from build123d import *

# Parameters (mm, degrees)
SKETCH1_W           = 50.8
SKETCH1_H           = 34.925
BOSS_EXTRUDE1_DEPTH = 1.27
SKETCH2_W           = 1.27
SKETCH2_H           = 34.925
BOSS_EXTRUDE2_DEPTH = 36.83
SKETCH3_R           = 2.0828
CUT_EXTRUDE1_DEPTH  = 36.83
SKETCH4_R           = 2.0828
CUT_EXTRUDE2_DEPTH  = 36.83


with BuildPart() as part:
    # Sketch1 → Boss-Extrude1 (new body)
    with BuildSketch(Plane.XY):
        Rectangle(SKETCH1_W, SKETCH1_H)
    extrude(amount=BOSS_EXTRUDE1_DEPTH)

    # Sketch2 → Boss-Extrude2 (add)
    with BuildSketch(Plane.XY.offset(1.27)):
        with Locations((-24.765, 0)):
            Rectangle(SKETCH2_W, SKETCH2_H)
    extrude(amount=BOSS_EXTRUDE2_DEPTH)

    # Sketch3 → Cut-Extrude1 (cut)
    with BuildSketch(Plane(origin=(-24.13, 0, 0), x_dir=(0, 0, -1), z_dir=(1, 0, 0))):
        with Locations((-10.4775, 8.73125)):
            Circle(SKETCH3_R)
        with Locations((-28.8925, -8.73125)):
            Circle(SKETCH3_R)
    extrude(amount=-CUT_EXTRUDE1_DEPTH, mode=Mode.SUBTRACT)

    # Sketch4 → Cut-Extrude2 (cut)
    with BuildSketch(Plane.XY.offset(1.27)):
        with Locations((-11.7475, 8.47725)):
            Circle(SKETCH4_R)
        with Locations((13.0175, -8.73125)):
            Circle(SKETCH4_R)
    extrude(amount=-CUT_EXTRUDE2_DEPTH, mode=Mode.SUBTRACT)


solid = part.part
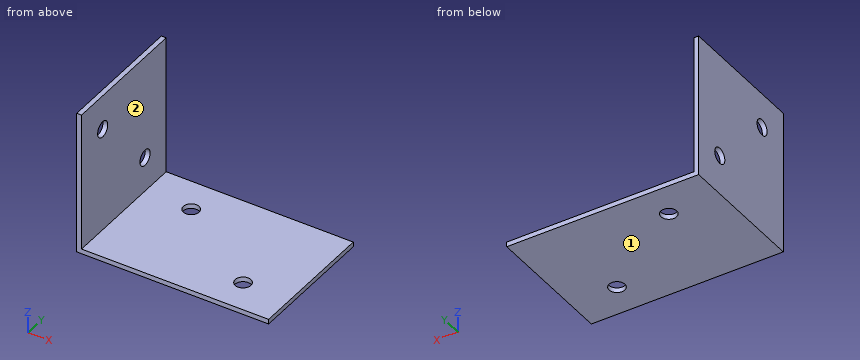
Model file for the job. Use its own axes, mm. Face numbers are marked on the shaded views. A direction names the side the tool comes from. Give positions to 0.01 mm unless a question says otherwise; leave off trailing zeros. Order: outer loops, then holes, each group sorted by start corner. A loop starts at its lowest first (then second) coordinate and runs counter-clockwise, first axis right, second up. Notation, with made-up numbers: (18, 74.5) - (72, 74.5) arc R24 ccw to (72, 107.5) - close; hole circle Ø2 at (20.5, 49.25). An arc over 180 degrees is marked (long way). One line per item, written item: value.
Item 1: Slice it at C-C (y = 5). List the corners of the cut face in (x, z).
Response values:
outline: (-25.4, 0) - (25.4, 0) - (25.4, 1.27) - (-24.13, 1.27) - (-24.13, 38.1) - (-25.4, 38.1) - close
Item 2: Slice it at D-D (z = 18). List the corners of the cut face in (x, y), then the cut area to 3 significant figures.
Response values:
outline: (-25.4, -17.46) - (-24.13, -17.46) - (-24.13, 17.46) - (-25.4, 17.46) - close
area: 44.4 mm2
Item 3: Pin check, flat tips, straight feed: pin 1 Ø3.5 at (y, z) = (-8.73, 28.89) entering from +X; pin 2 Ø12 at (x, z) = (8, 6.5) entering from +Y; pin 3 Ø2 at (x, y) = (-1, 8.5) entering from +Z; pin 4 Ø10.5 at (y, z) = (-2, 19.5) entering from +X. Stop position of each tip, or through.
Response values:
pin 1: through
pin 2: y = 17.46
pin 3: z = 1.27
pin 4: x = -24.13
Item 4: Slice it at B-B (x = 12). List the corners of the cut face in (y, z), then the cut area to 3 significant figures.
Response values:
outline: (-17.46, 0) - (-10.55, 0) - (-10.55, 1.27) - (-17.46, 1.27) - close; (-6.91, 0) - (17.46, 0) - (17.46, 1.27) - (-6.91, 1.27) - close
area: 39.7 mm2
Item 5: Tool access for the marked faces 1 and 2: list every direction of +Z, -Z, +X, -X, +Y, -Y with a clear straight run to the whole face (end or side of a thin tool).
Response values:
face 1: -Z, +X, -X, +Y, -Y
face 2: +Z, +X, +Y, -Y
Item 6: Slice it at A-A (z = 29.5). List the corners of the cut face in (x, y), then the cut area to 3 significant figures.
Response values:
outline: (-25.4, -17.46) - (-24.13, -17.46) - (-24.13, -10.72) - (-25.4, -10.72) - close; (-25.4, -6.74) - (-24.13, -6.74) - (-24.13, 17.46) - (-25.4, 17.46) - close
area: 39.3 mm2
Item 7: Wall check: line 1 (X direction, y = -1.5, z = 12); line 2 (Z direction, x = 6.5, y = -6.5). Give the ranges that are in metal, low to high.
Response values:
line 1: -25.4 to -24.13
line 2: 0 to 1.27
